Source: CAD feature listing. Evaluate the final solid. Frame: model axes, mm. A direction names the side the tool comes from. Round coordinates to 2 decimals unless told otherwise and drop trailing zeros. Loops run counter-clockwise (first coordinate to the right, second up) from the corner with the lowest first, then second, coordinate; pieces in that order, holes last.
Item 1: Pull-direction query (X, two-part tool) for faces 1 (the flat face through (-9, 17.12, -19)), 2 (the cylindrical face through (43.723, 3.039, -21.231)), 3 (the cylindrical face through (-1.256, 14.299, 28.547)); classes: released by +X, released by -X, zero draft, split by the parting line, or undercut.
Item 2: Section query A-A on y = 9.25. Return loops of the section in (x, z), then the cut area to 3 significant figures.
Item 3: First-contact query: P1, Ø4, axis at y = 7.5, z = 36, coming from the +X side; P2, Ø3, axis at y = 12.5, z = -29.5, coming from the -X side; P3, Ø3.5, axis at x = 21.18, z = -58.19, coming from the -Y side; P4, Ø6, axis at x = -35, z = 47.5, coming from the +Y side. Flat tips, straight axial feed; report the tip coordinate or a pass-through.
Item 4: Access query for faces 4 (the cylindrical face through (-15.49, 3.04, -36.98)), 5 (the flat face through (-25, 11.557, 15)). Directions: +Z, -Z, +X, -X, +Y, -Y. A direction counts if a zero-diameter tool reaches every point of the face in a straight line with its end or side. Return the directions, or none.
Item 5: Ray query, L1, parallel to Y at x = -20.5, z = 27; L2, parallel to Y at x = 20, z = 21; L3, parallel to X at y = 13.5, z = 0 (3 decimals). Return the intervals inside material, ascending.
```python
from build123d import *

# Parameters (mm, degrees)
SKETCH1_R           = 71.374
BOSS_EXTRUDE1_DEPTH = 5.9944
SKETCH2_R           = 28.575
SKETCH2_R_2         = 20.6502
BOSS_EXTRUDE2_DEPTH = 11.1252
CUT_EXTRUDE2_START  = -3.175
SKETCH3_R           = 20.6502
CUT_EXTRUDE2_DEPTH  = 3.175
SKETCH4_R           = 16.51
CUT_EXTRUDE3_DEPTH  = 102.946022345
SKETCH5_R           = 5.08
CUT_EXTRUDE4_DEPTH  = 102.549327063
SKETCH7_R           = 33.02
SKETCH7_R_2         = 28.575
BOSS_EXTRUDE3_DEPTH = 5.5626
SKETCH8_R           = 1.4478
CUT_EXTRUDE7_DEPTH  = 102.549327063
SKETCH9_R           = 5.08
CUT_EXTRUDE8_DEPTH  = 102.549327063


with BuildPart() as part:
    # Sketch1 → Boss-Extrude1 (new body)
    with BuildSketch(Plane(origin=(0, 0, 0), x_dir=(1, 0, 0), z_dir=(0, 1, 0))):
        with Locations(Location((0, 0, 0), (0, 0, 90))):
            Circle(SKETCH1_R)
    extrude(amount=BOSS_EXTRUDE1_DEPTH)

    # Sketch2 → Boss-Extrude2 (add)
    with BuildSketch(Plane(origin=(0, 5.9944, 0), x_dir=(1, 0, 0), z_dir=(0, 1, 0))):
        with Locations(Location((0, 0, 0), (0, 0, 90))):
            Circle(SKETCH2_R)
        with Locations(Location((0, 0, 0), (0, 0, 90))):
            Circle(SKETCH2_R_2, mode=Mode.SUBTRACT)
    extrude(amount=BOSS_EXTRUDE2_DEPTH)

    # Sketch3 → Cut-Extrude2 (cut)
    with BuildSketch(Plane(origin=(0, 5.9944, 0), x_dir=(1, 0, 0), z_dir=(0, 1, 0)).offset(CUT_EXTRUDE2_START)):
        with Locations(Location((0, 0, 0), (0, 0, 90))):
            Circle(SKETCH3_R)
    extrude(amount=CUT_EXTRUDE2_DEPTH, mode=Mode.SUBTRACT)

    # Sketch4 → Cut-Extrude3 (cut, through all)
    with BuildSketch(Plane(origin=(0, 2.8194, 0), x_dir=(1, 0, 0), z_dir=(0, 1, 0))):
        with Locations(Location((0, 0, 0), (0, 0, 270))):
            Circle(SKETCH4_R)
    extrude(amount=-CUT_EXTRUDE3_DEPTH, mode=Mode.SUBTRACT)

    # Sketch5 → Cut-Extrude4 (cut, through all)
    with BuildSketch(Plane(origin=(0, 5.9944, 0), x_dir=(1, 0, 0), z_dir=(0, 1, 0))):
        with Locations(Location((16.413387891, 40.624560588, 0), (0, 0, 270))):
            Circle(SKETCH5_R)
        with Locations(Location((26.975207541, -34.526691169, 0), (0, 0, 270))):
            Circle(SKETCH5_R)
        with Locations(Location((-1.529121448, -43.788309086, 0), (0, 0, 270))):
            Circle(SKETCH5_R)
        with Locations(Location((-29.317957518, -32.560890528, 0), (0, 0, 270))):
            Circle(SKETCH5_R)
        with Locations(Location((-43.388595432, -6.097869419, 0), (0, 0, 270))):
            Circle(SKETCH5_R)
        with Locations(Location((-37.157227333, 23.218412562, 0), (0, 0, 270))):
            Circle(SKETCH5_R)
        with Locations(Location((-13.539579609, 41.670541261, 0), (0, 0, 270))):
            Circle(SKETCH5_R)
    extrude(amount=-CUT_EXTRUDE4_DEPTH, mode=Mode.SUBTRACT)

    # Sketch7 → Boss-Extrude3 (add)
    with BuildSketch(Plane(origin=(0, 5.9944, 0), x_dir=(1, 0, 0), z_dir=(0, 1, 0))):
        with Locations(Location((0, 0, 0), (0, 0, 90))):
            Circle(SKETCH7_R)
        with Locations(Location((0, 0, 0), (0, 0, 90))):
            Circle(SKETCH7_R_2, mode=Mode.SUBTRACT)
    extrude(amount=BOSS_EXTRUDE3_DEPTH)

    # Sketch8 → Cut-Extrude7 (cut, through all)
    with BuildSketch(Plane(origin=(0, 5.9944, 0), x_dir=(1, 0, 0), z_dir=(0, 1, 0))):
        with Locations(Location((-53.628796334, 30.9626, 0), (0, 0, 270))):
            Circle(SKETCH8_R)
        with Locations(Location((-47.437455349, 39.804751287, 0), (0, 0, 270))):
            Circle(SKETCH8_R)
        with Locations(Location((-39.804751287, 47.437455349, 0), (0, 0, 270))):
            Circle(SKETCH8_R)
        with Locations(Location((-30.9626, 53.628796334, 0), (0, 0, 270))):
            Circle(SKETCH8_R)
        with Locations(Location((-21.179665779, 58.190653481, 0), (0, 0, 270))):
            Circle(SKETCH8_R)
        with Locations(Location((-10.753198132, 60.984417067, 0), (0, 0, 270))):
            Circle(SKETCH8_R)
        with Locations(Location((0, 61.9252, 0), (0, 0, 270))):
            Circle(SKETCH8_R)
        with Locations(Location((10.753198132, 60.984417067, 0), (0, 0, 270))):
            Circle(SKETCH8_R)
        with Locations(Location((21.179665779, 58.190653481, 0), (0, 0, 270))):
            Circle(SKETCH8_R)
        with Locations(Location((30.9626, 53.628796334, 0), (0, 0, 270))):
            Circle(SKETCH8_R)
        with Locations(Location((39.804751287, 47.437455349, 0), (0, 0, 270))):
            Circle(SKETCH8_R)
        with Locations(Location((47.437455349, 39.804751287, 0), (0, 0, 270))):
            Circle(SKETCH8_R)
        with Locations(Location((53.628796334, 30.9626, 0), (0, 0, 270))):
            Circle(SKETCH8_R)
        with Locations(Location((58.190653481, 21.179665779, 0), (0, 0, 270))):
            Circle(SKETCH8_R)
        with Locations(Location((60.984417067, 10.753198132, 0), (0, 0, 270))):
            Circle(SKETCH8_R)
        with Locations(Location((61.9252, 0, 0), (0, 0, 270))):
            Circle(SKETCH8_R)
        with Locations(Location((60.984417067, -10.753198132, 0), (0, 0, 270))):
            Circle(SKETCH8_R)
        with Locations(Location((58.190653481, -21.179665779, 0), (0, 0, 270))):
            Circle(SKETCH8_R)
        with Locations(Location((53.628796334, -30.9626, 0), (0, 0, 270))):
            Circle(SKETCH8_R)
        with Locations(Location((47.437455349, -39.804751287, 0), (0, 0, 270))):
            Circle(SKETCH8_R)
        with Locations(Location((39.804751287, -47.437455349, 0), (0, 0, 270))):
            Circle(SKETCH8_R)
        with Locations(Location((30.9626, -53.628796334, 0), (0, 0, 270))):
            Circle(SKETCH8_R)
        with Locations(Location((21.179665779, -58.190653481, 0), (0, 0, 270))):
            Circle(SKETCH8_R)
        with Locations(Location((10.753198132, -60.984417067, 0), (0, 0, 270))):
            Circle(SKETCH8_R)
        with Locations(Location((0, -61.9252, 0), (0, 0, 270))):
            Circle(SKETCH8_R)
        with Locations(Location((-10.753198132, -60.984417067, 0), (0, 0, 270))):
            Circle(SKETCH8_R)
        with Locations(Location((-21.179665779, -58.190653481, 0), (0, 0, 270))):
            Circle(SKETCH8_R)
        with Locations(Location((-30.9626, -53.628796334, 0), (0, 0, 270))):
            Circle(SKETCH8_R)
        with Locations(Location((-39.804751287, -47.437455349, 0), (0, 0, 270))):
            Circle(SKETCH8_R)
        with Locations(Location((-47.437455349, -39.804751287, 0), (0, 0, 270))):
            Circle(SKETCH8_R)
        with Locations(Location((-53.628796334, -30.9626, 0), (0, 0, 270))):
            Circle(SKETCH8_R)
        with Locations(Location((-58.190653481, -21.179665779, 0), (0, 0, 270))):
            Circle(SKETCH8_R)
        with Locations(Location((-60.984417067, -10.753198132, 0), (0, 0, 270))):
            Circle(SKETCH8_R)
        with Locations(Location((-61.9252, 0, 0), (0, 0, 270))):
            Circle(SKETCH8_R)
        with Locations(Location((-60.984417067, 10.753198132, 0), (0, 0, 270))):
            Circle(SKETCH8_R)
        with Locations(Location((-58.190653481, 21.179665779, 0), (0, 0, 270))):
            Circle(SKETCH8_R)
    extrude(amount=-CUT_EXTRUDE7_DEPTH, mode=Mode.SUBTRACT)

    # Sketch9 → Cut-Extrude8 (cut, through all)
    with BuildSketch(Plane(origin=(0, 5.9944, 0), x_dir=(1, 0, 0), z_dir=(0, 1, 0))):
        with Locations(Location((38.686348781, 20.569896523, 0), (0, 0, 270))):
            Circle(SKETCH9_R)
        with Locations(Location((42.857537126, -9.109650733, 0), (0, 0, 270))):
            Circle(SKETCH9_R)
    extrude(amount=-CUT_EXTRUDE8_DEPTH, mode=Mode.SUBTRACT)


solid = part.part
```
Data:
1. face 1: zero draft
1. face 2: undercut
1. face 3: split by the parting line
2. outline: circle Ø66.04 at (0, 0); hole circle Ø41.3 at (0, 0)
2. area: 2,090 mm2
3. P1: stops at x = 62.38
3. P2: stops at x = -16.96
3. P3: stops at y = 0
3. P4: stops at y = 5.99
4. face 4: +Y, -Y
4. face 5: +Y
5. L1: y = 0 to 5.99
5. L2: y = 0 to 11.56
5. L3: x = -28.575 to -20.65, 20.65 to 28.575
